Here's how the part is built. I have some questions about the finished solid (model axes, mm). Face numbers are marked on the shaded views. A direction names the side the tool comes from. Round coordinates to 2 decimals unless told otherwise and drop trailing zeros. Order: outer loops, then holes, each group sorted by start corner. A loop starts at its lowest first (then second) coordinate and runs counter-clockwise, first axis right, second up. Notation, with made-up numbers: M 2.5,83 L 61.5,83 A26 ccw 61.5,102 Z; hole C 58.25,-21.75 d1. An arc over 180 degrees is marked long. Use one line per item in the form item = value. Start each with the question number.
```python
from build123d import *

# Parameters (mm, degrees)
SKETCH_1_R          = 2.5
EXTRUDE_1_DEPTH     = 3.5
SKETCH_2_R          = 4.5
EXTRUDE_2_DEPTH     = 1.2
SKETCH_4_W          = 2.2
SKETCH_4_H          = 2.2
CUT_EXTRUDE_1_DEPTH = 2
FILLET_1_R          = 0.5


with BuildPart() as part:
    # 草图1 → 凸台-拉伸1 (new body)
    with BuildSketch(Plane(origin=(0, 0, 0), x_dir=(1, 0, 0), z_dir=(0, 1, 0))):
        with Locations(Location((0, 0, 0), (0, 0, 270))):
            Circle(SKETCH_1_R)
    extrude(amount=EXTRUDE_1_DEPTH)

    # 草图2 → 凸台-拉伸2 (add)
    with BuildSketch(Plane(origin=(0, 3.5, 0), x_dir=(1, 0, 0), z_dir=(0, 1, 0))):
        with Locations(Location((0.094879954, 0.012027373, 0), (0, 0, 270))):
            Circle(SKETCH_2_R)
    extrude(amount=EXTRUDE_2_DEPTH)

    # 草图4 → 切除-拉伸1 (cut)
    with BuildSketch(Plane(origin=(0, 4.7, 0), x_dir=(1, 0, 0), z_dir=(0, 1, 0))):
        Rectangle(SKETCH_4_W, SKETCH_4_H)
    extrude(amount=-CUT_EXTRUDE_1_DEPTH, mode=Mode.SUBTRACT)

    # 圆角1
    fillet_1_edges = [part.edges().sort_by_distance(p)[0] for p in [
        (0, 0, -2.5),
    ]]
    fillet(fillet_1_edges, radius=FILLET_1_R)


solid = part.part
```
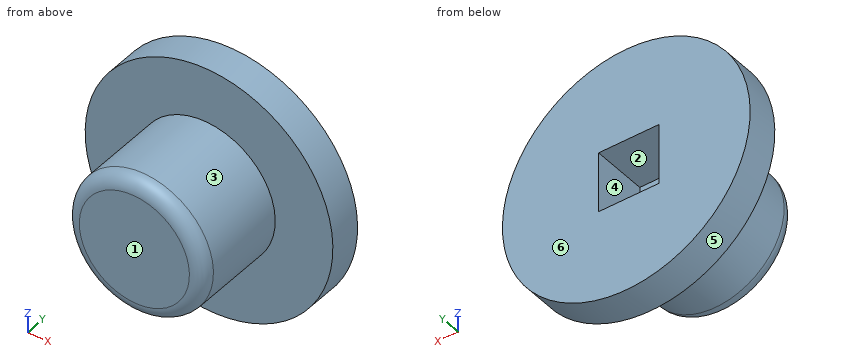
1) If we section it at D-D on x = -2.75: Write out the boundary of the cut face in (y, z).
2) On a 3-axis mill with a long thin cutter (end or side, diameter ignored), from which of +Z, -Z, +X, -X, +Y, -Y can I reach the whole of each face in a straight line? I mean the marked faces 1, 2 and 3. Say none if no direction works.
3) If we mould it in two halves opening along X, with no side actions, what happens to the marked faces 4, 5 and 6? For each: +X half, -X half, draft (parallel to the pull), parting line (faces both ways), or undercut.
4) Will these pins go through, and if not, where does the flat tip stop? pin 1 Ø0.6 at (x, y) = (-0.5, 3.5) entering from -Z; pin 2 Ø0.6 at (y, z) = (3.5, 0.5) entering from +X; pin 3 Ø0.6 at (y, z) = (4, -0.5) entering from -X.
5) If I drill on line 1 (Y direction, x = 3.5, z = 0); line 2 (X direction, y = 4, z = 0.5); line 3 (Z direction, x = 1.5, y = 2.55), over which ranges is the centre line in solid material (lowest first)?
6) If we section it at C-C on y = 3.8: Write out the boundary of the cut face in (x, z).
7) If we section it at A-A on z = 0: Write out the boundary of the cut face in (x, y).
8) If we section it at B-B on y = 2.35: Write out the boundary of the cut face in (x, z), then the cut area to 3 significant figures.
Completed:
q1.outline = M 3.5,-3.5 L 4.7,-3.5 L 4.7,3.47 L 3.5,3.47 Z
q2.face_1 = +Z, -Z, +X, -X, -Y
q2.face_2 = +Y
q2.face_3 = -Y
q3.face_4 = undercut
q3.face_5 = parting line
q3.face_6 = draft
q4.pin_1 = -4.5
q4.pin_2 = 4.59
q4.pin_3 = -4.4
q5.line_1 = 3.5 to 4.7
q5.line_2 = -4.38 to -1.1, 1.1 to 4.57
q5.line_3 = -2 to 2
q6.outline = C 0.09,-0.01 d9; hole M -1.1,-1.1 L 1.1,-1.1 L 1.1,1.1 L -1.1,1.1 Z
q7.outline = M -4.41,3.5 L -2.5,3.5 L -2.5,0.5 A0.5 ccw -2,0 L 2,0 A0.5 ccw 2.5,0.5 L 2.5,3.5 L 4.59,3.5 L 4.59,4.7 L 1.1,4.7 L 1.1,2.7 L -1.1,2.7 L -1.1,4.7 L -4.41,4.7 Z
q8.outline = C 0,0 d5
q8.area = 19.6 mm²
